Autodesk Inventor part; units mm, degrees
ref_plane "Work Plane1" through (40.64, 102.235, 6.35) normal (1, 0, 0) x (0, 0, -1)
ref_plane "YZ Plane" through (0, 0, 0) normal (1, 0, 0) x (0, 1, 0)
ref_plane "XZ Plane" through (0, 0, 0) normal (0, 1, 0) x (-1, 0, 0)
sketch "Sketch1" plane through (0, 0, 0) normal (0, 0, 1) x (1, 0, 0)
  line L0 (0, 0) -> (81.28, 0)
  line L1 (81.28, 0) -> (81.28, 152.4)
  line L2 (81.28, 152.4) -> (0, 152.4)
  line L3 (0, 152.4) -> (0, 0)
  line L4 (8.89, 21.59) -> (72.39, 21.59)
  line L5 (72.39, 21.59) -> (72.39, 130.81)
  line L6 (72.39, 130.81) -> (8.89, 130.81)
  line L7 (8.89, 130.81) -> (8.89, 21.59)
  dimension "d0" = 81.28
  dimension "d1" = 152.4
  dimension "d2" = 21.59
  dimension "d3" = 8.89
  dimension "d4" = 63.5
  dimension "d5" = 109.22
extrude "Extrusion1" add sketch "Sketch1" along normal blind 6.35
sketch "Sketch2" plane through (0, 0, 6.35) normal (0, 0, 1) x (1, 0, 0)
  line L0 (0, 0) -> (81.28, 0)
  line L1 (81.28, 0) -> (81.28, 152.4)
  line L2 (81.28, 152.4) -> (0, 152.4)
  line L3 (0, 152.4) -> (0, 0)
  line L4 (2.54, 2.54) -> (78.74, 2.54)
  line L5 (78.74, 2.54) -> (78.74, 149.86)
  line L6 (78.74, 149.86) -> (2.54, 149.86)
  line L7 (2.54, 149.86) -> (2.54, 2.54)
  dimension "d8" = 2.54
  dimension "d9" = 2.54
  dimension "d10" = 76.2
  dimension "d11" = 147.32
extrude "Extrusion2" add sketch "Sketch2" along normal blind 11.684
sketch "Sketch3" plane through (0, 0, 18.034) normal (0, 0, 1) x (1, 0, 0)
  line L0 (0, 0) -> (81.28, 0)
  line L1 (2.54, 2.54) -> (78.74, 2.54)
  line L2 (34.29, 0) -> (46.99, 0)
  line L3 (46.99, 0) -> (46.99, 2.54)
  line L4 (46.99, 2.54) -> (34.29, 2.54)
  line L5 (34.29, 2.54) -> (34.29, 0)
  line L6 (81.28, 0) -> (81.28, 152.4)
  line L7 (81.28, 152.4) -> (0, 152.4)
  line L8 (78.74, 2.54) -> (78.74, 149.86)
  line L9 (81.28, 121.285) -> (78.74, 121.285)
  line L10 (78.74, 121.285) -> (78.74, 102.235)
  line L11 (78.74, 102.235) -> (81.28, 102.235)
  line L12 (81.28, 102.235) -> (81.28, 121.285)
  dimension "d14" = 34.29
  dimension "d15" = 12.7
  dimension "d16" = 31.115
  dimension "d17" = 19.05
extrude "Extrusion3" cut sketch "Sketch3" against normal blind 11.684 contours L5 L1 L3 L0 | L11 L8 L9 L6
fillet "Fillet1" radius 6.35 1 edges at (78.74, 149.86, 12.192)
fillet "Fillet2" radius 6.35 3 edges at (2.54, 149.86, 12.192) (2.54, 2.54, 12.192) (78.74, 2.54, 12.192)
fillet "Fillet3" radius 6.35 4 edges at (81.28, 0, 9.017) (0, 0, 9.017) (81.28, 152.4, 9.017) (0, 152.4, 9.017)
sketch "Sketch4" plane through (0, 0, 0) normal (0, 0, -1) x (-1, 0, 0)
  line L0 (-46.99, 0) -> (-34.29, 0)
  arc A0 (-37.465, -19.05) -> (-34.29, 0) centre (-72.232, -3.4659) ccw
  arc A1 (-46.99, 0) -> (-43.815, -19.05) centre (-9.048, -3.4659) ccw
  line L1 (-6.35, 0) -> (-34.29, 0)
  line L2 (-6.35, 0) -> (-74.93, 0)
  arc A2 (-34.29, -19.05) -> (-31.75, 0) centre (-69.5649, -4.6523) ccw
  arc A3 (-49.53, 0) -> (-46.6296, -19.05) centre (-11.6381, -3.9766) ccw
  line L3 (-34.29, -19.05) -> (-37.465, -19.05)
  line L4 (-46.6296, -19.05) -> (-43.815, -19.05)
  point P0 (0, 0)
  dimension "d24" = 19.05
  dimension "d25" = 3.175
  dimension "d26" = 3.175
  dimension "d27" = 38.1
  dimension "d28" = 38.1
  dimension "d29" = 2.54
  dimension "d30" = 2.54
  dimension "d31" = 38.1
  dimension "d32" = 38.1
  dimension "d33" = 3.175
extrude "Extrusion4" add sketch "Sketch4" against normal blind 18.034
fillet "Fillet4" radius 6.35 1 edges at (31.75, 0, 9.017)
fillet "Fillet5" radius 6.35 1 edges at (49.53, 0, 9.017)
sketch "Sketch5" plane through (0, 0, 0) normal (0, 0, -1) x (-1, 0, 0)
  arc A0 (-35.9722, -19.0303) -> (-32.9017, 0) centre (-116.0568, 3.6542) ccw
  arc A1 (-49.1616, 0) -> (-45.6026, -19.0303) centre (-4.2841, -1.455) ccw
  arc A2 (-32.9017, 0) -> (-49.1616, 0) centre (-41.0317, -15.216) ccw
  line L0 (-35.9722, -19.0303) -> (-45.6026, -19.0303)
  line L1 (-46.6296, -19.05) -> (-43.815, -19.05)
  point P0 (0, 0)
extrude "Extrusion5" add sketch "Sketch5" against normal blind 6.35
sketch "Sketch6" plane through (0, 0, 6.35) normal (0, 0, 1) x (1, 0, 0)
  line L0 (74.93, 152.4) -> (6.35, 152.4)
  line L1 (6.35, 0) -> (25.1473, 0)
  line L2 (0, 146.05) -> (0, 6.35)
  point P0 (0, 0)
  point P1 (19.05, 10.795)
  point P2 (19.05, 141.605)
  dimension "d40" = 10.795
  dimension "d41" = 10.795
  dimension "d42" = 19.05
  dimension "d43" = 19.05
hole "Hole1" at (19.05, 10.795, 6.35) at (19.05, 141.605, 6.35) direction (0, 0, -1) diameter 3.683 depth 25.4 tip angle 118
sketch "Sketch7" plane through (0, 0, 6.35) normal (0, 0, 1) x (1, 0, 0)
  circle A0 centre (19.05, 10.795) radius 1.8415
  circle A1 centre (19.05, 10.795) radius 3.4925
  circle A2 centre (19.05, 141.605) radius 1.8415
  circle A3 centre (19.05, 141.605) radius 3.4925
  point P0 (0, 0)
  dimension "d51" = 6.985
  dimension "d52" = 6.985
extrude "Extrusion6" cut sketch "Sketch7" against normal blind 2.54
ref_plane "Work Plane1" through (40.64, 102.235, 6.35) normal (1, 0, 0) x (0, 0, -1)
mirror "Mirror1" about plane through (40.64, 102.235, 6.35) normal (1, 0, 0) of "Extrusion6", "Hole1"
equation "\"d26\" = d25"
equation "\"d28\" = d27"
equation "\"d30\" = d29"
properties part number "DS Phone Holder"
The model under review builds one solid part; all positions refer to its coordinate system, in mm. A direction names the side the tool comes from. Coordinates: 2 decimals unless noted, no trailing zeros. Write each loop counter-clockwise with the first axis right and the second up, starting at its lowest first coordinate (ties: lowest second). Pieces come first, ordered by that corner, then holes. Notation, with made-up numbers: (52, -5.75) -> (69, -5.75) arc R20 ccw to (69, 6.25) -> close; hole circle Ø2 at (-12, 5.25). An arc over 180 degrees is marked (long way). One line per item, written item: value. Start each with the question number.
Q1. Add section A-A, the plane x = 62.23. Give the boundary of the cut face in (y, z).
Q2. The part is to be moulded in two halves that separate along Y. For faces 1 (the face through (65.72, 10.64, 5.1)), 2 (the face through (20.171, 143.066, 1.878)), 3 (the face through (41, 152.4, 9)), 4 (the face through (79.37, 1.81, 9.14)), say which applies: +Y half, -Y half, draft (parallel to the pull), parting line (faces both ways), or undercut.
Q3. Add section B-B, the plane y = 93. Give the boundary of the cut face in (x, z), then the cut area to 3 significant figures.
Q4. Clearance check with flat-ended pins moving along their axes: P1, Ø3.5, axis at x = 20, y = 142, coming from the +Z side; P2, Ø3, axis at x = 62.23, y = 10.795, coming from the +Z side; P3, Ø5.5, axis at x = 18, z = 12, coming from the -Y side; P4, Ø0.8, axis at x = 80, z = 11.5, coming from the +Y side. State where each tip first meets the part, or that it passes through.
Q5. For faces 5 (the face through (29.6, -1.82, 9.14)), 6 (the face through (65.72, 141.45, 5.1)), 7 (the face through (41, 130.81, 3)), list the 3-axis set-ups (+Z, -Z, +X, -X, +Y, -Y) from which the entire face can be reached by the end or side of a thin tool; tool diameter is ignored.
Q6. To check wall thickness, follow probe 1 along Y at (x, z) = (19.05, 2.15); probe 2 along X at (y, z) = (122, 2); probe 3 along X at (y, z) = (21.5, 13). State the ranges of each line that lie inside material, in increasing order.
Q7. Add section D-D, the plane x = 54. Give the boundary of the cut face in (y, z), then the cut area to 3 significant figures.
Response:
1. outline: (0, 0) -> (8.95, 0) -> (8.95, 3.81) -> (7.3, 3.81) -> (7.3, 6.35) -> (2.54, 6.35) -> (2.54, 18.03) -> (0, 18.03) -> close; (12.64, 0) -> (21.59, 0) -> (21.59, 6.35) -> (14.29, 6.35) -> (14.29, 3.81) -> (12.64, 3.81) -> close; (130.81, 0) -> (139.76, 0) -> (139.76, 3.81) -> (138.11, 3.81) -> (138.11, 6.35) -> (130.81, 6.35) -> close; (143.45, 0) -> (152.4, 0) -> (152.4, 18.03) -> (149.86, 18.03) -> (149.86, 6.35) -> (145.1, 6.35) -> (145.1, 3.81) -> (143.45, 3.81) -> close
2. face 1: undercut
2. face 2: undercut
2. face 3: +Y half
2. face 4: -Y half
3. outline: (0, 0) -> (8.89, 0) -> (8.89, 6.35) -> (2.54, 6.35) -> (2.54, 18.03) -> (0, 18.03) -> close; (72.39, 0) -> (81.28, 0) -> (81.28, 18.03) -> (78.74, 18.03) -> (78.74, 6.35) -> (72.39, 6.35) -> close
3. area: 172 mm²
4. P1: z = 3.81
4. P2: through
4. P3: y = 0
4. P4: y = 150.35
5. face 5: +Z, -Z, -X, -Y
5. face 6: +Z
5. face 7: +Z, -Z
6. probe 1: 0 to 8.95, 12.64 to 21.59, 130.81 to 139.76, 143.45 to 152.4
6. probe 2: 0 to 8.89, 72.39 to 81.28
6. probe 3: 0 to 2.54, 78.74 to 81.28
7. outline: (-0.33, 0) -> (21.59, 0) -> (21.59, 6.35) -> (2.54, 6.35) -> (2.54, 18.03) -> (-0.33, 18.03) -> close; (130.81, 0) -> (152.4, 0) -> (152.4, 18.03) -> (149.86, 18.03) -> (149.86, 6.35) -> (130.81, 6.35) -> close
7. area: 340 mm²
